Here's how the part is built. I have some questions about the finished solid (model axes, mm). Coordinates: 2 decimals unless noted, no trailing zeros. Loops run counter-clockwise (first coordinate to the right, second up) from the corner with the lowest first, then second, coordinate; pieces in that order, holes last. Notation, with made-up numbers: (-29, 50.5) - (-17, 50.5) arc R17 ccw to (-17, 76.5) - close; hole circle Ø6 at (-25.75, 40.5). An arc over 180 degrees is marked (long way). Use a Markdown table: item, result.
Autodesk Inventor part; units mm, degrees
ref_plane "YZ Plane" through (0, 0, 0) normal (1, 0, 0) x (0, 1, 0)
ref_plane "XZ Plane" through (0, 0, 0) normal (0, 1, 0) x (-1, 0, 0)
ref_plane "XY Plane" through (0, 0, 0) normal (0, 0, 1) x (1, 0, 0)
sketch "Sketch1" plane through (0, 0, 0) normal (1, 0, 0) x (0, 1, 0)
  line L0 (0, 0) -> (4.7625, 0)
  line L1 (4.7625, 0) -> (4.7625, -150.4315)
  line L2 (4.7625, -150.4315) -> (0, -150.4315)
  line L3 (0, -150.4315) -> (0, 0)
  dimension "d1" = 4.7625
  dimension "d2" = 150.4315
extrude "Extrusion1" add sketch "Sketch1" along normal blind 0.7937
sketch "Sketch2" plane through (0, 0, -150.4315) normal (0, 0, -1) x (-1, 0, 0)
  line L0 (-0.7937, 0) -> (-0.7937, 4.7625)
  line L1 (-0.7937, 0) -> (71.5963, 0)
  line L2 (71.5963, 0) -> (71.5963, 4.7625)
  line L3 (71.5963, 4.7625) -> (-0.7937, 4.7625)
  line L4 (-0.7937, 4.7625) -> (-0.7937, 0)
  point P0 (0, 0)
  dimension "d5" = 72.39
  dimension "d6" = 4.7625
extrude "Extrusion2" add sketch "Sketch2" against normal blind 0.7937
sketch "Sketch3" plane through (-71.5963, 0, -150.4315) normal (-1, 0, 0) x (0, 0, 1)
  line L0 (150.4315, 4.7625) -> (150.4315, 0)
  line L1 (0, 0) -> (150.4315, 0)
  line L2 (150.4315, 0) -> (150.4315, 4.7625)
  line L3 (150.4315, 4.7625) -> (0, 4.7625)
  line L4 (0, 4.7625) -> (0, 0)
extrude "Extrusion3" add sketch "Sketch3" against normal blind 0.7937
sketch "Sketch4" plane through (-71.5963, 0, 0) normal (0, 0, 1) x (1, 0, 0)
  line L0 (0, 0) -> (0, 4.7625)
  line L1 (71.5963, 4.7625) -> (72.39, 4.7625)
  line L2 (0, 0) -> (72.39, 0)
  line L3 (72.39, 0) -> (72.39, 4.7625)
  line L4 (72.39, 4.7625) -> (0, 4.7625)
  line L5 (0, 4.7625) -> (0, 0)
  point P0 (71.5963, 0)
  point P1 (71.5963, 4.7625)
extrude "Extrusion4" add sketch "Sketch4" against normal blind 0.7937
sketch "Sketch5" plane through (0.7937, 0, 0) normal (0, 0, 1) x (1, 0, 0)
  circle A0 centre (-36.195, 2.3813) radius 2.2098
extrude "Extrusion5" cut sketch "Sketch5" against normal blind 0.7937
sketch "Sketch6" plane through (0.7937, 0, -150.4315) normal (0, 0, -1) x (-1, 0, 0)
  circle A0 centre (36.195, 2.3813) radius 2.2098
  point P0 (0, 0)
  point P1 (72.39, 0)
extrude "Extrusion6" cut sketch "Sketch6" against normal blind 0.7937
properties part number "Back rubber bands"
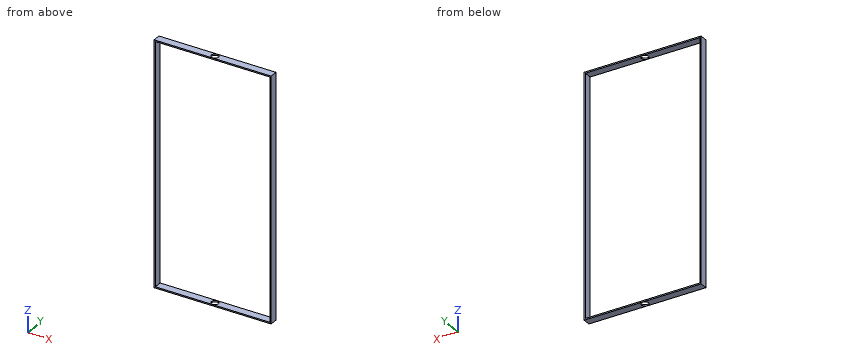
Q1. I want a section at C-C, the plane y = 1.5. Write out the boundary of the cut face in (x, z), then the cut area to 3 significant figures.
Check values:
| item | result |
|---|---|
| outline | (-71.6, -150.43) - (-37.43, -150.43) - (-37.43, -149.64) - (-70.8, -149.64) - (-70.8, -0.79) - (-37.43, -0.79) - (-37.43, 0) - (-71.6, 0) - close; (-33.37, -150.43) - (0.79, -150.43) - (0.79, 0) - (-33.37, 0) - (-33.37, -0.79) - (0, -0.79) - (0, -149.64) - (-33.37, -149.64) - close |
| area | 345 mm^2 |
Q2. Will this pin go through, and if not, where does the flat tip stop? P1, Ø2.5, axis at x = -35.4, y = 2.38, coming from the -Z side.
Check values:
| item | result |
|---|---|
| P1 | through |
Q3. I want a section at A-A, the plane x = -43. Write out the boundary of the cut face in (y, z), then the cut area to 3 significant figures.
Check values:
| item | result |
|---|---|
| outline | (0, -150.43) - (4.76, -150.43) - (4.76, -149.64) - (0, -149.64) - close; (0, -0.79) - (4.76, -0.79) - (4.76, 0) - (0, 0) - close |
| area | 7.56 mm^2 |
Q4. Please list where these lines run through material, in increasing order: L1, parallel to X at y = 2.2, z = -50; L2, parallel to Z at x = -61, y = 3.3. Write a range as from..to.
Check values:
| item | result |
|---|---|
| L1 | -71.6..-70.8, 0..0.79 |
| L2 | -150.43..-149.64, -0.79..0 |
Q5. I want a section at B-B, the plane z = -79.5. Write out the boundary of the cut face in (x, y).
Check values:
| item | result |
|---|---|
| outline | (-71.6, 0) - (-70.8, 0) - (-70.8, 4.76) - (-71.6, 4.76) - close; (0, 0) - (0.79, 0) - (0.79, 4.76) - (0, 4.76) - close |
